Verification items for this drawing (mm, ordinates from the low corner). A direction names the side the tool comes from. Give positions to 0.01 mm unless a question says otherwise; leave off trailing zeros. Loops run counter-clockwise (first coordinate to the right, second up) from the corner with the lowest first, then second, coordinate; pieces in that order, holes last. Notation, with made-up numbers: (83, 26) -> (131, 26) arc R15 ccw to (131, 31) -> close; hole circle Ø6 at (-35, -27.75). An arc over 180 degrees is marked (long way). Answer in a Markdown table with one row per item. Add a question column.
Q1. Gauge pin test, flat ends, axial feed: P1, Ø10, axis at y = 73, z = 43, coming from the +X side; P2, Ø5, axis at y = 69.5, z = 11.5, coming from the -X side; P3, Ø22, axis at y = 76, z = 31, coming from the -X side. Record the tip position at first contact, or that the pin passes through.
Q2. Release check for a two-part mould opening along X. For the marked faces 4, 5 and 6 record: pulls with the +X half, pulls with the -X half, needs draft (parallel to the pull), parting line crosses it, or undercut.
Q3. Section check C-C on z = 25. Enter the section's corners in (x, y), and give its area (3 significant figures).
Q4. Set-up check for the marked faces 1, 2 and 3: record each of +Z, -Z, +X, -X, +Y, -Y from which the full face is reachable in a straight line by a thin tool's end or side.
Q5. Section check D-D on y = 34.5. Enter the section's corners in (x, z).
Q6. Section check A-A on x = 48. Enter the section's corners in (y, z), and give its area (3 significant figures).
Q7. Material ranges on probe 1 along Y at (x, z) = (47, 36); probe 2 along Y at (x, z) = (10.5, 11.5); probe 3 along X at (y, z) = (46, 20), recorded low to high.
Q8. Section check B-B on y = 12. Enter the section's corners in (x, z), and give its area (3 significant figures).
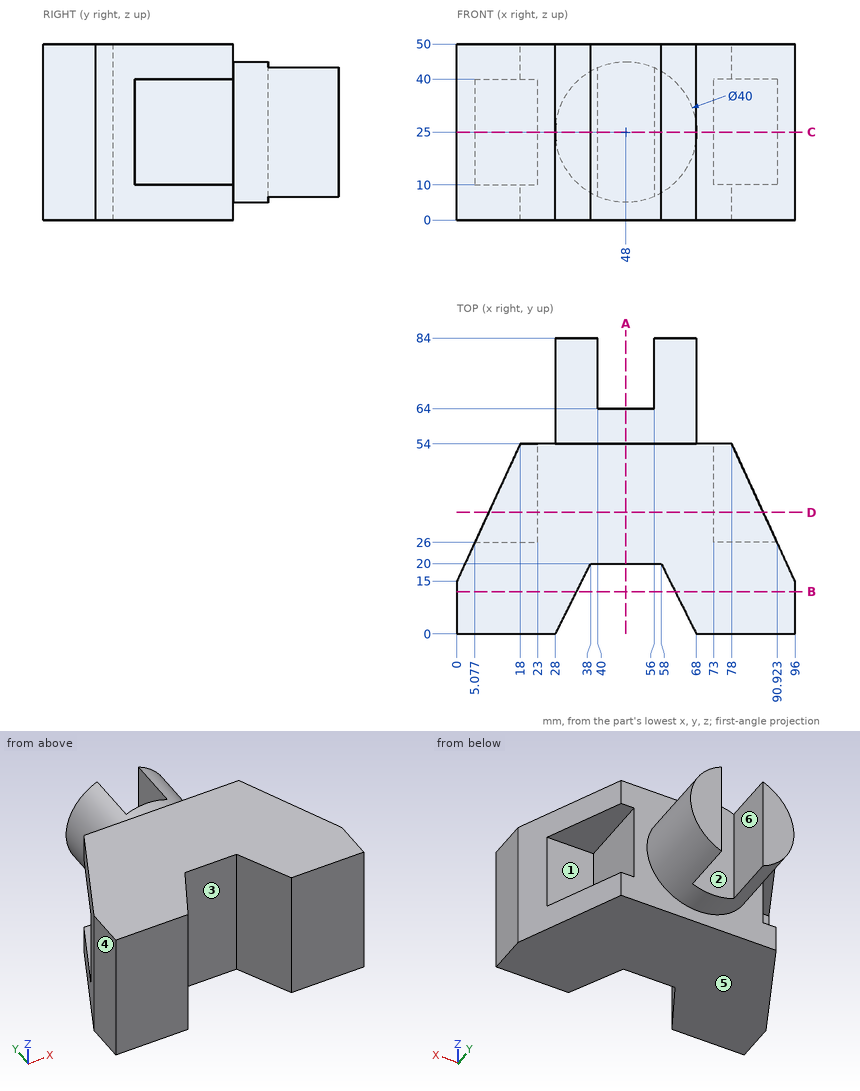
Taken from the geometry:
| question | item | result |
|---|---|---|
| 1 | P1 | stops at x = 63.2 |
| 1 | P2 | stops at x = 31.3 |
| 1 | P3 | stops at x = 28 |
| 2 | face 4 | pulls with the -X half |
| 2 | face 5 | needs draft |
| 2 | face 6 | undercut |
| 3 | outline | (0, 0) -> (28, 0) -> (38, 20) -> (58, 20) -> (68, 0) -> (96, 0) -> (96, 15) -> (90.92, 26) -> (73, 26) -> (73, 54) -> (68, 54) -> (68, 84) -> (56, 84) -> (56, 64) -> (40, 64) -> (40, 84) -> (28, 84) -> (28, 54) -> (23, 54) -> (23, 26) -> (5.08, 26) -> (0, 15) -> close |
| 3 | area | 4,120 mm² |
| 4 | face 1 | +X, +Y |
| 4 | face 2 | +Z, -Z, +Y |
| 4 | face 3 | +Z, -Z, -Y |
| 5 | outline | (9, 0) -> (87, 0) -> (87, 10) -> (73, 10) -> (73, 40) -> (87, 40) -> (87, 50) -> (9, 50) -> (9, 40) -> (23, 40) -> (23, 10) -> (9, 10) -> close |
| 6 | outline | (20, 0) -> (54, 0) -> (54, 5) -> (64, 5) -> (64, 45) -> (54, 45) -> (54, 50) -> (20, 50) -> close |
| 6 | area | 2,100 mm² |
| 7 | probe 1 | y = 20 to 64 |
| 7 | probe 2 | y = 0 to 26 |
| 7 | probe 3 | x = 23 to 73 |
| 8 | outline | (0, 0) -> (34, 0) -> (34, 50) -> (0, 50) -> close; (62, 0) -> (96, 0) -> (96, 50) -> (62, 50) -> close |
| 8 | area | 3,400 mm² |
